Verification items for the finished model (mm, model axes). Coordinates: 2 decimals unless noted, no trailing zeros. Order: outer loops, then holes, each group sorted by start corner. A loop starts at its lowest first (then second) coordinate and runs counter-clockwise, first axis right, second up. Notation, with made-up numbers: M 40.25,-17 L 79.25,-17 A13 ccw 79.25,-1 Z; hole C 4.5,-29.5 d4. An arc over 180 degrees is marked long. Return JSON: item names as keys, results as strings. Group by question number.
1. Gauge pin test, flat end, axial feed: pin 1 (3.5 mm diameter, centred on x = 85.025, z = -4, fed in from -Y). Record the tip position at first contact, or that the pin passes through.
2. Section check A-A, the plane z = -52. Record the cut outline in (x, y) (3 decimals).
3. Section check C-C, the plane y = 1. Give the number of separate pieces and of enclosed holes in the cut face, plus the area to 3 significant figures.
4. Section check B-B, the plane x = 75.5. Record the cut outline in (y, z).
5. Material ranges on line 1 along Z through (x, y) = (77, 0.45); line 2 along X through (y, z) = (0.8, -303.5) (3 decimals); line 3 along Z through (x, y) = (4.2, 0.6), recorded low to high.
```python
from build123d import *

# Parameters (mm, degrees)
SKETCH1_W              = 89.225
SKETCH1_H              = 307.5
SKETCH1_W_2            = 69.225
SKETCH1_H_2            = 51
BOSS_EXTRUDE1_DEPTH    = 2
M2_5_CLEARANCE_HOLE6_D = 2.9


with BuildPart() as part:
    # Sketch1 → Boss-Extrude1 (new body)
    with BuildSketch(Plane(origin=(0, 0, 0), x_dir=(1, 0, 0), z_dir=(0, 1, 0))):
        with Locations((44.6125, 153.75)):
            Rectangle(SKETCH1_W, SKETCH1_H)
        Polygon((10, 10), (79.225, 10), (79.225, 21.8), (79.225, 81.2), (79.225, 101.2), (10, 101.2), (10, 81.2), (10, 21.8), align=None, mode=Mode.SUBTRACT)
        with Locations((44.6125, 142.7)):
            Rectangle(SKETCH1_W_2, SKETCH1_H_2, mode=Mode.SUBTRACT)
        Polygon((10, 297.5), (79.225, 297.5), (79.225, 283.2), (79.225, 209.2), (79.225, 184.2), (10, 184.2), (10, 209.2), (10, 283.2), align=None, mode=Mode.SUBTRACT)
    extrude(amount=BOSS_EXTRUDE1_DEPTH)

    # M2.5 Clearance Hole6 (through all)
    with Locations(Plane(origin=(0, 2, 0), x_dir=(1, 0, 0), z_dir=(0, 1, 0))):
        with Locations((85.025, 4), (4.2, 4), (4.2, 109.2), (4.2, 176.2), (4.2, 303.5), (85.025, 303.5), (85.025, 176.2), (85.025, 109.2)):
            Hole(M2_5_CLEARANCE_HOLE6_D / 2)


solid = part.part
```
Answers follow:
{
 "1": {"pin 1": "y = 0"},
 "2": {"outline": "M 0,0 L 10,0 L 10,2 L 0,2 Z; M 79.225,0 L 89.225,0 L 89.225,2 L 79.225,2 Z"},
 "3": {"separate pieces": "1", "enclosed holes": "11", "area": "9,700 mm^2"},
 "4": {"outline": "M 0,-307.5 L 2,-307.5 L 2,-297.5 L 0,-297.5 Z; M 0,-184.2 L 2,-184.2 L 2,-168.2 L 0,-168.2 Z; M 0,-117.2 L 2,-117.2 L 2,-101.2 L 0,-101.2 Z; M 0,-10 L 2,-10 L 2,0 L 0,0 Z"},
 "5": {"line 1": "-307.5 to -297.5, -184.2 to -168.2, -117.2 to -101.2, -10 to 0", "line 2": "0 to 2.75, 5.65 to 83.575, 86.475 to 89.225", "line 3": "-307.5 to -304.95, -302.05 to -177.65, -174.75 to -110.65, -107.75 to -5.45, -2.55 to 0"}
}
